```python
from build123d import *

# Parameters (mm, degrees)
RESSALTO_EXTRUS_O2_DEPTH        = 5.5
ESBO_O3_OUTSIDE_W               = 115.272
ESBO_O3_OUTSIDE_H               = 113.576
ESBO_O3_OUTSIDE_R               = 5.5
CORTE_EXTRUS_O1_DEPTH           = 13
CORTE_EXTRUS_O1_DRAFT           = -75
ESBO_O4_OUTSIDE_W               = 115.272
ESBO_O4_OUTSIDE_H               = 113.576
ESBO_O4_OUTSIDE_R               = 5.5
CORTE_EXTRUS_O2_DEPTH           = 13
CORTE_EXTRUS_O2_DRAFT           = -75
FURO_ROSCADO_DE_M61_D           = 5
FURO_ROSCADO_DE_M61_CSINK_D     = 6.05
FURO_ROSCADO_DE_M61_CSINK_ANGLE = 90
CHANFRO1_SIZE                   = 0.5


with BuildPart() as part:
    # Esboço2 → Ressalto-extrusão2 (new body)
    with BuildSketch(Plane.XY):
        Polygon((3.180933655, 5.496816753), (-3.169916121, 5.503177729), (-6.350849776, 0.006360976), (-3.180933655, -5.496816753), (3.169916121, -5.503177729), (6.350849776, -0.006360976), align=None)
    extrude(amount=RESSALTO_EXTRUS_O2_DEPTH)


with BuildPart() as corte_extrus_o1_tool:
    # Esboço3 outside → Corte-extrusão1 (with draft: the straight prism first)
    with BuildSketch(Plane.XY.offset(5.5)):
        Rectangle(ESBO_O3_OUTSIDE_W, ESBO_O3_OUTSIDE_H)
        Circle(ESBO_O3_OUTSIDE_R, mode=Mode.SUBTRACT)
    extrude(amount=-CORTE_EXTRUS_O1_DEPTH)
    # Corte-extrusão1: the draft: its side faces are tilted about the plane it starts from
    corte_extrus_o1_sides = [corte_extrus_o1_tool.faces().sort_by_distance(p)[0] for p in [
        (0, -56.788, -1),
        (57.636, 0, -1),
        (0, 56.788, -1),
        (-57.636, 0, -1),
        (-5.5, 0, -1),
    ]]
    draft(corte_extrus_o1_sides, Plane.XY.offset(5.5), CORTE_EXTRUS_O1_DRAFT)


with BuildPart() as part_1:
    add(part.part)

    # Corte-extrusão1: cut by corte_extrus_o1_tool
    add(corte_extrus_o1_tool.part, mode=Mode.SUBTRACT)


with BuildPart() as corte_extrus_o2_tool:
    # Esboço4 outside → Corte-extrusão2 (with draft: the straight prism first)
    with BuildSketch(Plane(origin=(0, 0, 0), x_dir=(-1, 0, 0), z_dir=(0, 0, -1))):
        Rectangle(ESBO_O4_OUTSIDE_W, ESBO_O4_OUTSIDE_H)
        Circle(ESBO_O4_OUTSIDE_R, mode=Mode.SUBTRACT)
    extrude(amount=-CORTE_EXTRUS_O2_DEPTH)
    # Corte-extrusão2: the draft: its side faces are tilted about the plane it starts from
    corte_extrus_o2_sides = [corte_extrus_o2_tool.faces().sort_by_distance(p)[0] for p in [
        (0, -56.788, 6.5),
        (-57.636, 0, 6.5),
        (0, 56.788, 6.5),
        (57.636, 0, 6.5),
        (5.5, 0, 6.5),
    ]]
    draft(corte_extrus_o2_sides, Plane(origin=(0, 0, 0), x_dir=(-1, 0, 0), z_dir=(0, 0, -1)), CORTE_EXTRUS_O2_DRAFT)


with BuildPart() as part_2:
    add(part_1.part)

    # Corte-extrusão2: cut by corte_extrus_o2_tool
    add(corte_extrus_o2_tool.part, mode=Mode.SUBTRACT)

    # Furo roscado de M61 (through all)
    with Locations(Plane(origin=(0, 0, 0), x_dir=(-1, 0, 0), z_dir=(0, 0, -1))):
        with Locations((0, 0)):
            CounterSinkHole(FURO_ROSCADO_DE_M61_D / 2, FURO_ROSCADO_DE_M61_CSINK_D / 2, counter_sink_angle=FURO_ROSCADO_DE_M61_CSINK_ANGLE)

    # Chanfro1
    chanfro1_edges = [part_2.edges().sort_by_distance(p)[0] for p in [
        (-2.5, 0, 5.5),
    ]]
    chamfer(chanfro1_edges, length=CHANFRO1_SIZE)


solid = part_2.part
```
Design review of the part built by this model. Coordinates are the model's own, in mm. Coordinates: 2 decimals unless noted, no trailing zeros. Loops run counter-clockwise (first coordinate to the right, second up) from the corner with the lowest first, then second, coordinate; pieces in that order, holes last. Notation, with made-up numbers: (-30.5, 24.5) - (13.5, 24.5) arc R26 cw to (13.5, 53.5) - close; hole circle Ø2 at (64, 16). An arc over 180 degrees is marked (long way). Use CSV: the item, a comma, the result in double quotes. Start each with the question number.
1) Consider section A-A on z = 0.7. Write out the cut boundary in (x, y).
2) For pin 1 Ø3 at (x, z) = (-3.5, 5) entering from +Y, flat-tipped, find the tip position at first contact; note if it passes through.
3) Wall thickness on L1, parallel to Y at x = 0, z = 2.95; L2, parallel to X at y = 2.75, z = 2; L3, parallel to X at y = -2.25, z = 2.65: over which ranges is each line inside the solid? List them lowest first. Write a range as from..to.
Geometry says:
1,outline,"(-6.35, 0.01) - (-3.18, -5.5) - (3.17, -5.5) - (6.35, -0.01) - (3.18, 5.5) - (-3.17, 5.5) - close; hole circle Ø5 at (0, 0)"
2,pin 1,"y = 5.5"
3,L1,"-5.5..-2.5, 2.5..5.5"
3,L2,"-4.76..4.76"
3,L3,"-5.05..-1.09, 1.09..5.05"
